Could you check a few things on this drawing? It's one solid part, dimensions in mm from its lowest x, y, z. A direction names the side the tool comes from. Give positions to 0.01 mm unless a question says otherwise; leave off trailing zeros. Write each loop counter-clockwise with the first axis right and the second up, starting at its lowest first coordinate (ties: lowest second). Pieces come first, ordered by that corner, then holes. Notation, with made-up numbers: M 10.5,81 L 60.5,81 A21 ccw 60.5,95 Z; hole C 54,37.25 d7. An arc over 180 degrees is marked long. Write each question's results on one line, items separated by ' | '. Start each with the question number.
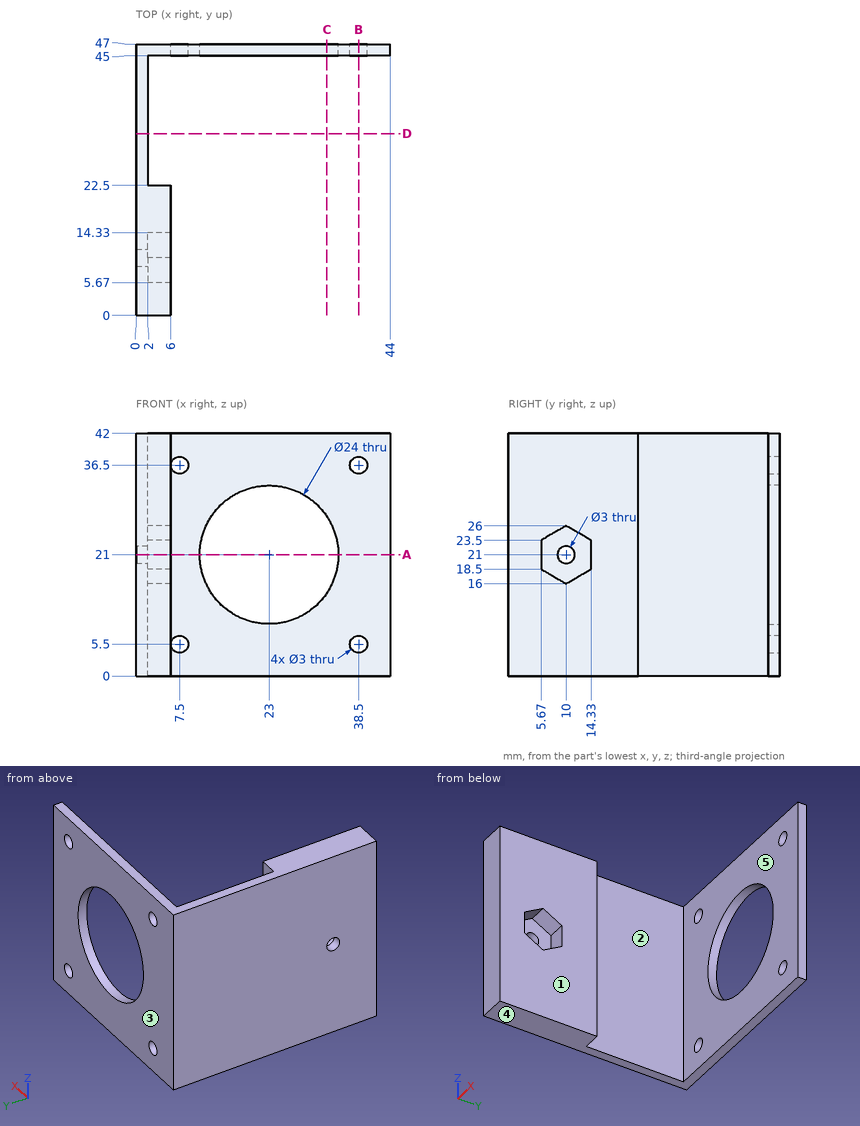
Q1. Please list where these lines run through material, in increasing order: line 1 (Z direction, x = 38.5, y = 45.75); line 2 (X direction, y = 46.2, z = 21); line 3 (X direction, y = 46, z = 36). Write a range as [from, to].
Q2. For the marked faces 4 and 5, which set-ups out of +Z, -Z, +X, -X, +Y, -Y let a thin tool reach every point of the face, with its end or its side?
Q3. If we section it at B-B (x = 38.5): Please give me the cut outline in (y, z), plus the area to 3 significant figures.
Q4. If we section it at A-A (z = 21): Please give me the cut outline in (x, y).
Q5. If we mould it in two halves opening along Y, with no side actions, what happens to the marked faces 1, 2 and 3? For each: pulls with the +Y half, pulls with the -Y half, needs draft (parallel to the pull), parting line crosses it, or undercut.
Q6. If we section it at C-C (x = 33): Please give me the cut outline in (y, z).
Q7. If we section it at D-D (y = 31.5): Please give me the cut outline in (x, z).
Q8. I'm going to push flat-ended pins straight in: P1, Ø5, axis at y = 26.5, z = 24.5, coming from the -X side; P2, Ø9.5, axis at y = 10.5, z = 23.5, coming from the +X side; P3, Ø1.5, axis at y = 30.5, z = 34.5, coming from the +X side; P4, Ø8, axis at x = 26.5, z = 4.5, coming from the -Y side. Where does each tip first touch, or does it pass through?
Determined:
1) line 1: z = [0, 4], [7, 35], [38, 42] | line 2: x = [0, 11], [35, 44] | line 3: x = [0, 6.09], [8.91, 37.09], [39.91, 44]
2) face 4: -Z, +X, -X, +Y, -Y | face 5: +Z, -Z, +X
3) outline: M 45,0 L 47,0 L 47,4 L 45,4 Z; M 45,7 L 47,7 L 47,35 L 45,35 Z; M 45,38 L 47,38 L 47,42 L 45,42 Z | area: 72.0 mm²
4) outline: M 0,0 L 6,0 L 6,5.67 L 2,5.67 L 2,8.5 L 0,8.5 Z; M 0,11.5 L 2,11.5 L 2,14.33 L 6,14.33 L 6,22.5 L 2,22.5 L 2,45 L 11,45 L 11,47 L 0,47 Z; M 35,45 L 44,45 L 44,47 L 35,47 Z
5) face 1: needs draft | face 2: undercut | face 3: pulls with the +Y half
6) outline: M 45,0 L 47,0 L 47,14.37 L 45,14.37 Z; M 45,27.63 L 47,27.63 L 47,42 L 45,42 Z
7) outline: M 0,0 L 2,0 L 2,42 L 0,42 Z
8) P1: stops at x = 0 | P2: stops at x = 6 | P3: stops at x = 2 | P4: stops at y = 45
